```python
from build123d import *

# Parameters (mm, degrees)
BOX049_W                    = 6
BOX049_H                    = 6
BOX049_DEPTH                = 2
BOX050_W                    = 6
BOX050_H                    = 6
BOX050_DEPTH                = 2
BOX050_PLACEMENT_ANGLE      = 135
BOX051_W                    = 6
BOX051_H                    = 6
BOX051_DEPTH                = 2
BOX052_W                    = 6
BOX052_H                    = 6
BOX052_DEPTH                = 2
BOX052_PLACEMENT_ANGLE      = 225
BOX053_W                    = 6
BOX053_H                    = 6
BOX053_DEPTH                = 2
BOX054_W                    = 6
BOX054_H                    = 6
BOX054_DEPTH                = 2
BOX054_PLACEMENT_ANGLE      = 45
BOX047_W                    = 6
BOX047_H                    = 6
BOX047_DEPTH                = 2
BOX048_W                    = 6
BOX048_H                    = 6
BOX048_DEPTH                = 2
BOX048_PLACEMENT_ANGLE      = 45
COMPOUND039_PLACEMENT_ANGLE = 22.5
CYLINDER112_R               = 1.5
CYLINDER112_DEPTH           = 15
CYLINDER112_PLACEMENT_ANGLE = 45
CYLINDER113_R               = 1.5
CYLINDER113_DEPTH           = 15
CYLINDER114_R               = 1.5
CYLINDER114_DEPTH           = 15
CYLINDER114_PLACEMENT_ANGLE = 135
CYLINDER115_R               = 1.5
CYLINDER115_DEPTH           = 15
CYLINDER116_R               = 1.5
CYLINDER116_DEPTH           = 15
CYLINDER116_PLACEMENT_ANGLE = 225
CYLINDER117_R               = 1.5
CYLINDER117_DEPTH           = 15
CYLINDER118_R               = 1.5
CYLINDER118_DEPTH           = 15
CYLINDER118_PLACEMENT_ANGLE = 45
CYLINDER111_R               = 1.5
CYLINDER111_DEPTH           = 15
COMPOUND897_PLACEMENT_ANGLE = 22.5
TUBE007_R                   = 29
TUBE007_R_2                 = 23
TUBE007_DEPTH               = 6


with BuildPart() as krychle049:
    # Box049 → Box049 (new body)
    with BuildSketch(Plane(origin=(-23, -3, -13), x_dir=(0, 1, 0), z_dir=(0, 0, 1))):
        with Locations((3, 3)):
            Rectangle(BOX049_W, BOX049_H)
    extrude(amount=BOX049_DEPTH)


with BuildPart() as krychle050:
    # Box050 → Box050 (new body)
    with BuildSketch(Plane.XY):
        with Locations((3, 3)):
            Rectangle(BOX050_W, BOX050_H)
    extrude(amount=BOX050_DEPTH)


with BuildPart() as krychle050_1:
    # Box050 placement: moved
    add(krychle050.part.moved(Location((-14.142136, -18.384776, -13))).rotate(Axis((-14.142136, -18.384776, -13), (0, 0, 1)), BOX050_PLACEMENT_ANGLE))


with BuildPart() as krychle051:
    # Box051 → Box051 (new body)
    with BuildSketch(Plane(origin=(3, -23, -13), x_dir=(-1, 0, 0), z_dir=(0, 0, 1))):
        with Locations((3, 3)):
            Rectangle(BOX051_W, BOX051_H)
    extrude(amount=BOX051_DEPTH)


with BuildPart() as krychle052:
    # Box052 → Box052 (new body)
    with BuildSketch(Plane.XY):
        with Locations((3, 3)):
            Rectangle(BOX052_W, BOX052_H)
    extrude(amount=BOX052_DEPTH)


with BuildPart() as krychle052_1:
    # Box052 placement: moved
    add(krychle052.part.moved(Location((18.384776, -14.142136, -13))).rotate(Axis((18.384776, -14.142136, -13), (0, 0, 1)), BOX052_PLACEMENT_ANGLE))


with BuildPart() as krychle053:
    # Box053 → Box053 (new body)
    with BuildSketch(Plane(origin=(23, 3, -13), x_dir=(0, -1, 0), z_dir=(0, 0, 1))):
        with Locations((3, 3)):
            Rectangle(BOX053_W, BOX053_H)
    extrude(amount=BOX053_DEPTH)


with BuildPart() as krychle054:
    # Box054 → Box054 (new body)
    with BuildSketch(Plane.XY):
        with Locations((3, 3)):
            Rectangle(BOX054_W, BOX054_H)
    extrude(amount=BOX054_DEPTH)


with BuildPart() as krychle054_1:
    # Box054 placement: moved
    add(krychle054.part.moved(Location((14.142136, 18.384776, -13))).rotate(Axis((14.142136, 18.384776, -13), (0, 0, -1)), BOX054_PLACEMENT_ANGLE))


with BuildPart() as krychle047:
    # Box047 → Box047 (new body)
    with BuildSketch(Plane(origin=(-3, 23, -13), x_dir=(1, 0, 0), z_dir=(0, 0, 1))):
        with Locations((3, 3)):
            Rectangle(BOX047_W, BOX047_H)
    extrude(amount=BOX047_DEPTH)


with BuildPart() as compound039:
    # Box048 → Box048 (new body)
    with BuildSketch(Plane.XY):
        with Locations((3, 3)):
            Rectangle(BOX048_W, BOX048_H)
    extrude(amount=BOX048_DEPTH)


with BuildPart() as compound039_1:
    # Box048 placement: moved
    add(compound039.part.moved(Location((-18.384776, 14.142136, -13))).rotate(Axis((-18.384776, 14.142136, -13), (0, 0, 1)), BOX048_PLACEMENT_ANGLE))

    # Compound039: union Krychle049, Krychle050, Krychle051, Krychle052, Krychle053, Krychle054, Krychle047
    add(krychle049.part)
    add(krychle050_1.part)
    add(krychle051.part)
    add(krychle052_1.part)
    add(krychle053.part)
    add(krychle054_1.part)
    add(krychle047.part)


with BuildPart() as compound039_2:
    # Compound039 placement: moved
    add(compound039_1.part.rotate(Axis((0, 0, 0), (0, 0, 1)), COMPOUND039_PLACEMENT_ANGLE))


with BuildPart() as obj1:
    # Cylinder112 → Cylinder112 (new body)
    with BuildSketch(Plane.XY):
        Circle(CYLINDER112_R)
    extrude(amount=CYLINDER112_DEPTH)


with BuildPart() as obj1_1:
    # Cylinder112 placement: moved
    add(obj1.part.moved(Location((-18.384776, 18.384776, -20))).rotate(Axis((-18.384776, 18.384776, -20), (0, 0, 1)), CYLINDER112_PLACEMENT_ANGLE))


with BuildPart() as obj2:
    # Cylinder113 → Cylinder113 (new body)
    with BuildSketch(Plane(origin=(-26, 0, -20), x_dir=(0, 1, 0), z_dir=(0, 0, 1))):
        Circle(CYLINDER113_R)
    extrude(amount=CYLINDER113_DEPTH)


with BuildPart() as obj3:
    # Cylinder114 → Cylinder114 (new body)
    with BuildSketch(Plane.XY):
        Circle(CYLINDER114_R)
    extrude(amount=CYLINDER114_DEPTH)


with BuildPart() as obj3_1:
    # Cylinder114 placement: moved
    add(obj3.part.moved(Location((-18.384776, -18.384776, -20))).rotate(Axis((-18.384776, -18.384776, -20), (0, 0, 1)), CYLINDER114_PLACEMENT_ANGLE))


with BuildPart() as obj4:
    # Cylinder115 → Cylinder115 (new body)
    with BuildSketch(Plane(origin=(0, -26, -20), x_dir=(-1, 0, 0), z_dir=(0, 0, 1))):
        Circle(CYLINDER115_R)
    extrude(amount=CYLINDER115_DEPTH)


with BuildPart() as obj5:
    # Cylinder116 → Cylinder116 (new body)
    with BuildSketch(Plane.XY):
        Circle(CYLINDER116_R)
    extrude(amount=CYLINDER116_DEPTH)


with BuildPart() as obj5_1:
    # Cylinder116 placement: moved
    add(obj5.part.moved(Location((18.384776, -18.384776, -20))).rotate(Axis((18.384776, -18.384776, -20), (0, 0, 1)), CYLINDER116_PLACEMENT_ANGLE))


with BuildPart() as obj6:
    # Cylinder117 → Cylinder117 (new body)
    with BuildSketch(Plane(origin=(26, 0, -20), x_dir=(0, -1, 0), z_dir=(0, 0, 1))):
        Circle(CYLINDER117_R)
    extrude(amount=CYLINDER117_DEPTH)


with BuildPart() as obj7:
    # Cylinder118 → Cylinder118 (new body)
    with BuildSketch(Plane.XY):
        Circle(CYLINDER118_R)
    extrude(amount=CYLINDER118_DEPTH)


with BuildPart() as obj7_1:
    # Cylinder118 placement: moved
    add(obj7.part.moved(Location((18.384776, 18.384776, -20))).rotate(Axis((18.384776, 18.384776, -20), (0, 0, -1)), CYLINDER118_PLACEMENT_ANGLE))


with BuildPart() as compound897:
    # Cylinder111 → Cylinder111 (new body)
    with BuildSketch(Plane(origin=(0, 26, -20), x_dir=(1, 0, 0), z_dir=(0, 0, 1))):
        Circle(CYLINDER111_R)
    extrude(amount=CYLINDER111_DEPTH)

    # Compound897: union obj1, obj2, obj3, obj4, obj5, obj6, obj7
    add(obj1_1.part)
    add(obj2.part)
    add(obj3_1.part)
    add(obj4.part)
    add(obj5_1.part)
    add(obj6.part)
    add(obj7_1.part)


with BuildPart() as compound897_1:
    # Compound897 placement: moved
    add(compound897.part.rotate(Axis((0, 0, 0), (0, 0, 1)), COMPOUND897_PLACEMENT_ANGLE))


with BuildPart() as cut311:
    # Tube007 → Tube007 (new body)
    with BuildSketch(Plane.XY.offset(-16)):
        Circle(TUBE007_R)
        Circle(TUBE007_R_2, mode=Mode.SUBTRACT)
    extrude(amount=TUBE007_DEPTH)

    # Cut532: cut Compound897
    add(compound897_1.part, mode=Mode.SUBTRACT)

    # Cut311: cut Compound039
    add(compound039_2.part, mode=Mode.SUBTRACT)


solid = cut311.part
```
Geometry check sheet. Reference: the model listing, model coordinates, mm. A direction names the side the tool comes from. Round coordinates to 2 decimals unless told otherwise and drop trailing zeros. Order: outer loops, then holes, each group sorted by start corner. A loop starts at its lowest first (then second) coordinate and runs counter-clockwise, first axis right, second up. Notation, with made-up numbers: (18, 46.25) - (25, 46.25) arc R9 ccw to (25, 62.25) - close; hole circle Ø11 at (-20.75, 11.5). An arc over 180 degrees is marked (long way). Use a Markdown table: item, result. Add a question column.
1) Set-up check for faces 1 (the flat face through (22.763, -12.676, -12.014)), 2 (the flat face through (-22.763, 12.676, -12.014)), 3 (the flat face through (-10, -26, -11)), 4 (the cylindrical face through (25.47, -10.34, -14.52)): record each of +Z, -Z, +X, -X, +Y, -Y from which the full face is reachable in a straight line by a thin tool's end or side.
2) Section check D-D (y = -7). Record the cut outline in (x, z).
3) Section check A-A (y = 0). Record the cut outline in (x, z), then the cut area to 3 significant figures.
4) Gauge pin test, flat ends, axial feed: P1, Ø2.5, axis at x = 24.02, y = 9.95, coming from the +Z side; P2, Ø2, axis at x = -16, z = -13.5, coming from the +Y side; P3, Ø1.5, axis at x = -20.5, z = -12, coming from the -Y side; P4, Ø3, axis at y = 22, z = -12.5, coming from the -X side. Record the tip position at first contact, or that the pin passes through.
5) Section check C-C (z = -14.85). Count the separate pieces of the cut face and the enclosed holes in it, then the cut area to 3 significant figures.
6) Mould release check, pull along Z, two halves, no side actions. Record for faces 5 (the flat face through (26, 10, -11)), 6 (the cylindrical face through (22.544, 9.69, -14.521)), 7 (the flat face through (-13, -19.2, -10)): released by +Z, released by -Z, zero draft, split by the parting line, or undercut.
7) Thickness scan on line 1 along Z through (x, y) = (26, -9); line 2 along X through (y, z) = (24.5, -14.65); line 3 along Y through (x, z) = (-25, -12.8). Record the ranges inside material, lowest first.
Established:
| question | item | result |
|---|---|---|
| 1 | face 1 | +X |
| 1 | face 2 | -X |
| 1 | face 3 | none |
| 1 | face 4 | +Z, -Z |
| 2 | outline | (-28.14, -16) - (-21.91, -16) - (-21.91, -10) - (-28.14, -10) - close; (21.91, -16) - (28.14, -16) - (28.14, -10) - (21.91, -10) - close; hole (-24.74, -13) - (-22, -13) - (-22, -11) - (-24.74, -11) - close; hole (22, -13) - (24.74, -13) - (24.74, -11) - (22, -11) - close |
| 3 | outline | (-29, -16) - (-23, -16) - (-23, -10) - (-29, -10) - close; (23, -16) - (29, -16) - (29, -10) - (23, -10) - close |
| 3 | area | 72.0 mm2 |
| 4 | P1 | through |
| 4 | P2 | y = 24.82 |
| 4 | P3 | y = -21.24 |
| 4 | P4 | x = -20.51 |
| 5 | separate pieces | 1 |
| 5 | enclosed holes | 9 |
| 5 | area | 924 mm2 |
| 6 | face 5 | undercut |
| 6 | face 6 | zero draft |
| 6 | face 7 | released by +Z |
| 7 | line 1 | -16 to -13, -11 to -10 |
| 7 | line 2 | -15.52 to -11.37, -8.53 to 8.53, 11.37 to 15.52 |
| 7 | line 3 | -14.7 to -13.6, -7.11 to 7.11, 13.6 to 14.7 |
